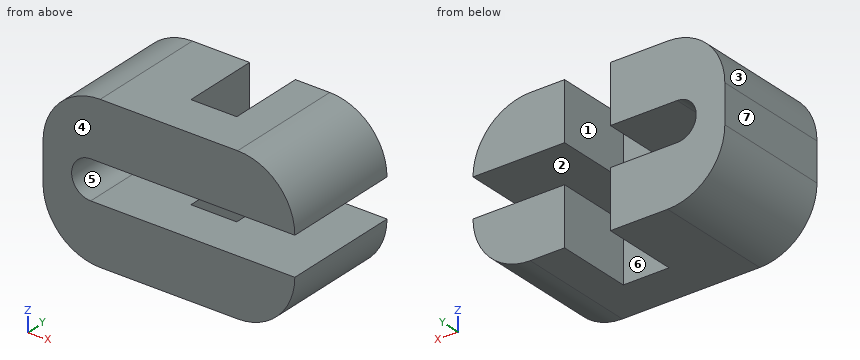
```python
from build123d import *

# Parameters (mm, degrees)
CROQUIS1_W              = 33
CROQUIS1_H              = 20
SALIENTE_EXTRUIR1_DEPTH = 15.7
CORTAR_EXTRUIR1_REACH   = 27.894
CROQUIS2_R              = 2.5
CROQUIS6_W              = 6
CROQUIS6_H              = 20
CORTAR_EXTRUIR2_DEPTH   = 10
CORTAR_EXTRUIR3_START   = -15.7
CROQUIS7_W              = 26.75
CROQUIS7_H              = 5
CORTAR_EXTRUIR3_DEPTH   = 15.7
REDONDEO1_R             = 7.5


with BuildPart() as part:
    # Croquis1 → Saliente-Extruir1 (new body)
    with BuildSketch(Plane(origin=(0, 0, 0), x_dir=(1, 0, 0), z_dir=(0, 1, 0))):
        with Locations((-1.5, 0)):
            Rectangle(CROQUIS1_W, CROQUIS1_H)
    extrude(amount=SALIENTE_EXTRUIR1_DEPTH)

    # Croquis2 → Cortar-Extruir1 (cut, up to next)
    with BuildSketch(Plane(origin=(0, 15.7, 0), x_dir=(1, 0, 0), z_dir=(0, 1, 0)), mode=Mode.PRIVATE) as cortar_extruir1_sk1:
        with Locations(Location((11.75, 0, 0), (0, 0, 270))):
            Circle(CROQUIS2_R)
    cortar_extruir1_tool1 = extrude(cortar_extruir1_sk1.sketch, amount=-CORTAR_EXTRUIR1_REACH, mode=Mode.PRIVATE) & part.part
    # Croquis2 → Cortar-Extruir1 (cut, up to next)
    with BuildSketch(Plane(origin=(0, 15.7, 0), x_dir=(1, 0, 0), z_dir=(0, 1, 0)), mode=Mode.PRIVATE) as cortar_extruir1_sk2:
        with Locations(Location((-11.75, 0, 0), (0, 0, 270))):
            Circle(CROQUIS2_R)
    cortar_extruir1_tool2 = extrude(cortar_extruir1_sk2.sketch, amount=-CORTAR_EXTRUIR1_REACH, mode=Mode.PRIVATE) & part.part
    add(cortar_extruir1_tool1.solids().sort_by_distance((11.75, 15.7, 0))[0], mode=Mode.SUBTRACT)
    add(cortar_extruir1_tool2.solids().sort_by_distance((-11.75, 15.7, 0))[0], mode=Mode.SUBTRACT)

    # Croquis6 → Cortar-Extruir2 (cut)
    with BuildSketch(Plane(origin=(0, 15.7, 0), x_dir=(1, 0, 0), z_dir=(0, 1, 0))):
        Rectangle(CROQUIS6_W, CROQUIS6_H)
    extrude(amount=-CORTAR_EXTRUIR2_DEPTH, mode=Mode.SUBTRACT)

    # Croquis7 → Cortar-Extruir3 (cut)
    with BuildSketch(Plane(origin=(0, 15.7, 0), x_dir=(1, 0, 0), z_dir=(0, 1, 0)).offset(CORTAR_EXTRUIR3_START)):
        with Locations((1.625, 0)):
            Rectangle(CROQUIS7_W, CROQUIS7_H)
    extrude(amount=CORTAR_EXTRUIR3_DEPTH, mode=Mode.SUBTRACT)

    # Redondeo1
    redondeo1_edges = [part.edges().sort_by_distance(p)[0] for p in [
        (-18, 7.85, -10),
        (-18, 7.85, 10),
        (15, 7.85, -10),
        (15, 7.85, 10),
    ]]
    fillet(redondeo1_edges, radius=REDONDEO1_R - 0.0001)  # a hair under: the kernel refuses the full size


solid = part.part
```
Read the model definition and answer for the solid it produces. Units are mm, in the model's axes. Face numbers are marked on the shaded views. A direction names the side the tool comes from. Coordinates: 2 decimals unless noted, no trailing zeros. Write each loop counter-clockwise with the first axis right and the second up, starting at its lowest first coordinate (ties: lowest second). Pieces come first, ordered by that corner, then holes. Notation, with made-up numbers: (-22.75, -4) -> (3.25, -4) arc R18 ccw to (3.25, 20) -> close; hole circle Ø5 at (73, -25.75). An arc over 180 degrees is marked (long way). Write item = value, one per line.
(1) Straight lines are drawn through the part: L1, parallel to Z at x = -4.5, y = 10; L2, parallel to Z at x = -14, y = 3.75; L3, parallel to Y at x = 2, z = 6.5. For each, find the intervals that lie inside material, in ascending order. Write a range as from..to.
From the geometry:
L1 = -10..-2.5, 2.5..10
L2 = -9.13..-1.09, 1.09..9.13
L3 = 0..5.7
(2) Given pin 1 Ø1 at (y, z) = (1.5, 0) entering from +X; pin 2 Ø8 at (y, z) = (10.5, 7.5) entering from -X; pin 3 Ø1.5 at (y, z) = (8.5, 1.5) entering from +X, each flat-ended and moving along its own axis, determine where each tip first touches the part or whether it passes through.
From the geometry:
pin_1 = -14.2
pin_2 = -17.93
pin_3 = -12.84
(3) Section D-D on z = 1.5 is taken. Write down the section's boundary in (x, y), plus the area to 3 significant figures.
From the geometry:
outline = (-18, 0) -> (-13.75, 0) -> (-13.75, 15.7) -> (-18, 15.7) -> close
area = 66.7 mm2
(4) For a pull along X with two mould halves and no side action, classify the marked faces 4, 5, 6 and 7 as +X half, -X half, draft (parallel to the pull), parting line (faces both ways), or undercut.
From the geometry:
face_4 = draft
face_5 = +X half
face_6 = undercut
face_7 = -X half
(5) Which of the six approach directions +Z, -Z, +X, -X, +Y, -Y give full straight-line access (tool end or side, diameter ignored) to the marked faces 1, 2 and 3?
From the geometry:
face_1 = +Z, -Z, +Y
face_2 = +X, +Y, -Y
face_3 = +Z, -X, +Y, -Y
(6) Section A-A on y = 6.25 is taken. Count the separate pieces of the cut face and the enclosed holes in it, plus the area to 3 significant figures.
From the geometry:
separate_pieces = 3
enclosed_holes = 0
area = 378 mm2
(7) Section B-B on x = 5.5 is taken. Write down the section's boundary in (y, z), plus the area to 4 significant figures.
From the geometry:
outline = (0, -10) -> (15.7, -10) -> (15.7, -2.5) -> (0, -2.5) -> close; (0, 2.5) -> (15.7, 2.5) -> (15.7, 10) -> (0, 10) -> close
area = 235.5 mm2
